Can you work these out from the model? Positions are in its coordinate system, mm. A direction names the side the tool comes from. Coordinates: 2 decimals unless noted, no trailing zeros. Loops run counter-clockwise (first coordinate to the right, second up) from the corner with the lowest first, then second, coordinate; pieces in that order, holes last.
```python
from build123d import *

# Parameters (mm, degrees)
SKETCH_1_W             = 30
SKETCH_1_H             = 20
EXTRUDE_1_DEPTH        = 223
CUT_EXTRUDE_1_DEPTH    = 225.396969677
HOLE_WIZARD_M5_1_D     = 4.2
HOLE_WIZARD_M5_1_DEPTH = 14
HOLE_WIZARD_M5_1_TIP   = 1.2618073
HOLE_WIZARD_M5_2_D     = 4.2


with BuildPart() as part:
    # 草图1 → 凸台-拉伸1 (new body)
    with BuildSketch(Plane(origin=(0, 0, 0), x_dir=(1, 0, 0), z_dir=(0, 1, 0))):
        Rectangle(SKETCH_1_W, SKETCH_1_H)
    extrude(amount=EXTRUDE_1_DEPTH)

    # 草图2 → 切除-拉伸1 (cut, through all)
    with BuildSketch(Plane.XY.offset(-10)):
        Polygon((7.168333691, 20), (-10, 20), (-10, 52.276467338), align=None)
        Polygon((10, 89.876467338), (-7.168333691, 57.6), (10, 25.323532662), align=None)
        Polygon((-10, 127.476467338), (-10, 62.923532662), (7.168333691, 95.2), align=None)
        Polygon((10, 165.076467338), (-7.168333691, 132.8), (10, 100.523532662), align=None)
        Polygon((-10, 202.676467338), (-10, 138.123532662), (7.168333691, 170.4), align=None)
        Polygon((-7.168333691, 208), (10, 208), (10, 175.723532662), align=None)
    extrude(amount=CUT_EXTRUDE_1_DEPTH, mode=Mode.SUBTRACT)

    # M5 螺纹孔1
    with Locations(Plane(origin=(0, 0, 0), x_dir=(-1, 0, 0), z_dir=(0, -1, 0))):
        with Locations((8, 0), (-8, 0)):
            Hole(HOLE_WIZARD_M5_1_D / 2, depth=HOLE_WIZARD_M5_1_DEPTH)
            with Locations((0, 0, -(HOLE_WIZARD_M5_1_DEPTH + HOLE_WIZARD_M5_1_TIP / 2))):  # 118° drill point
                Cone(0, HOLE_WIZARD_M5_1_D / 2, HOLE_WIZARD_M5_1_TIP, mode=Mode.SUBTRACT)

    # M5 螺纹孔2 (through all)
    with Locations(Plane(origin=(15, 0, 0), x_dir=(0, 0, -1), z_dir=(1, 0, 0))):
        with Locations((0, 215)):
            Hole(HOLE_WIZARD_M5_2_D / 2)


solid = part.part
```
Item 1: I need wall thicknesses on line 1 along X through (y, z) = (30.5, -2); line 2 along Z through (x, y) = (-3.5, 215); line 3 along X through (y, z) = (108.5, -7.75). Which ranges of each line are inside material? Lowest first, please.
Results are:
line 1: x = -15 to -10, 1.58 to 7.25, 10 to 15
line 2: z = -10 to -2.1, 2.1 to 10
line 3: x = -15 to -10, 0.09 to 5.76, 10 to 15
Item 2: I'm going to push a flat-ended pin straight in: P1, Ø3.5, axis at y = 215, z = 0, coming from the +X side. Where does the tip first touch, or does it pass through?
Results are:
P1: passes through
Item 3: Suppose I cut it at B-B, the plane x = -3.25. Count the separate pieces of the cut face and the enclosed holes in it, plus the area to 3 significant figures.
Results are:
separate pieces: 7
enclosed holes: 1
area: 1,750 mm2
Item 4: Suppose I cut it at C-C, the plane y = 145. Please give me the cut outline in (x, z), plus the area to 3 significant figures.
Results are:
outline: (-15, -10) - (-10, -10) - (-10, 10) - (-15, 10) - close; (-6.34, -10) - (-0.68, -10) - (-0.68, 10) - (-6.34, 10) - close; (10, -10) - (15, -10) - (15, 10) - (10, 10) - close
area: 313 mm2
Item 5: Suppose I cut it at A-A, the plane z = -4.5. Please give me the cut outline in (x, y), plus the area to 3 significant figures.
Results are:
outline: (-15, 0) - (15, 0) - (15, 223) - (-15, 223) - close; hole (-10, 20) - (7.17, 20) - (-10, 52.28) - close; hole (-10, 62.92) - (7.17, 95.2) - (-10, 127.48) - close; hole (-10, 138.12) - (7.17, 170.4) - (-10, 202.68) - close; hole (-7.17, 57.6) - (10, 25.32) - (10, 89.88) - close; hole (-7.17, 132.8) - (10, 100.52) - (10, 165.08) - close; hole (-7.17, 208) - (10, 175.72) - (10, 208) - close
area: 3,920 mm2
Item 6: On a 3-axis mill with a long thin cutter (end or side, diameter ignored), from which of +Z, -Z, +X, -X, +Y, -Y can I reach the whole of each face in a straight line? I mean faces 1 (the face through (-10.1, 7.1, -0.09)), 2 (the face through (0, 0, 0)), 3 (the face through (-10, 96, 0)). Say none if no direction works.
Results are:
face 1: -Y
face 2: +Z, -Z, +X, -X, -Y
face 3: +Z, -Z
Item 7: We'd pull the mould along Y, two halves only. Please class faces 4 (the face through (-10, 171, 0)), 5 (the face through (8.364, 15.043, -0.016)), 6 (the face through (-15, 110, 0)): +Y half, -Y half, draft (parallel to the pull), parting line (faces both ways), or undercut.
Results are:
face 4: undercut
face 5: -Y half
face 6: draft
